Verification items for this drawing (mm, ordinates from the low corner). Round coordinates to 2 decimals unless told otherwise and drop trailing zeros. Write each loop counter-clockwise with the first axis right and the second up, starting at its lowest first coordinate (ties: lowest second). Pieces come first, ordered by that corner, then holes. Notation, with made-up numbers: M 57.25,38 L 74.25,38 A20 ccw 74.25,66 Z; hole C -12.5,-21 d2. An arc over 180 degrees is marked long. Write each question's results on one line, items separated by ' | '.
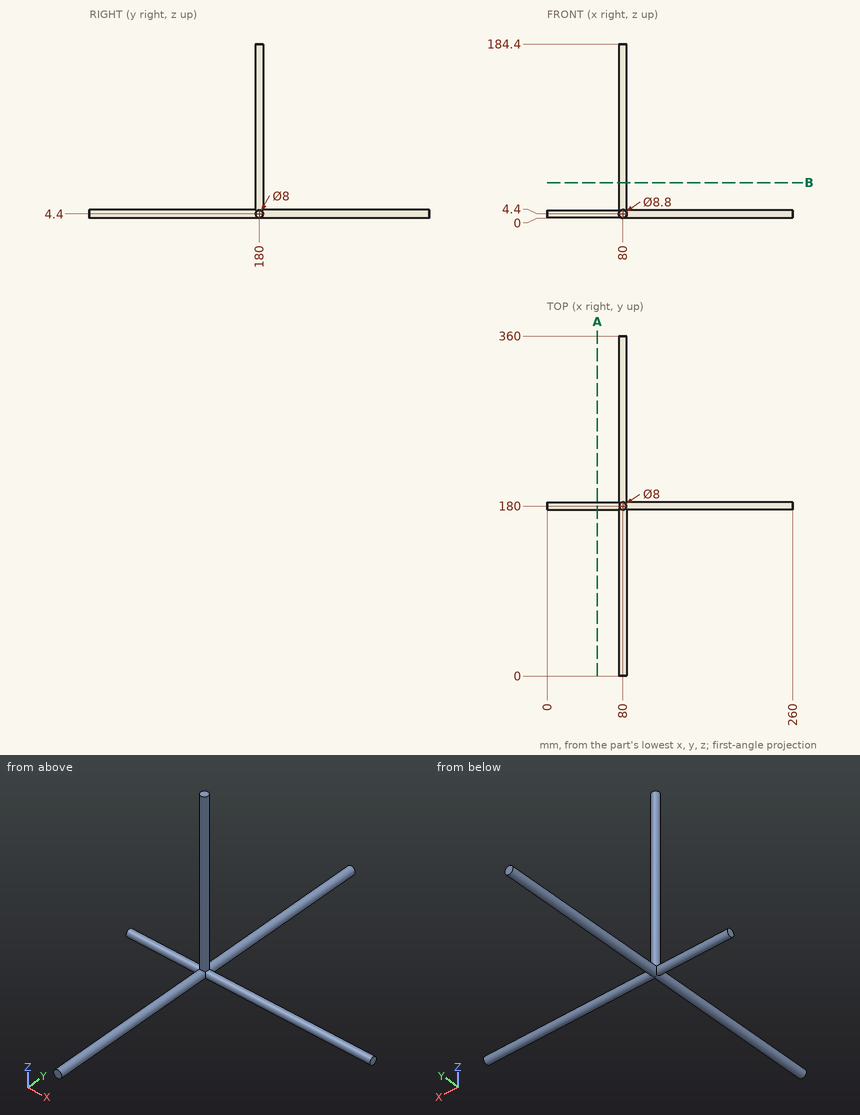
1) Sectioned sample at A-A, the plane x = 53. Record the cut outline in (y, z).
Calculated:
outline: C 180,4.4 d8
2) Material ranges on line 1 (X direction, y = 176.5, z = 92), recorded low to high. Write a range as [from, to].
Calculated:
line 1: x = [78.06, 81.94]
3) Sectioned sample at B-B, the plane z = 37.5. Record the cut outline in (x, y).
Calculated:
outline: C 80,180 d8
4) Depth check by flat-ended pin: P1, Ø1.5, axis at x = 231.5, y = 181.5, coming from the +Z side; P2, Ø10, axis at x = 189.5, y = 169, coming from the -Z side. Enter the tip coordinate at first touch or a pass-through.
Calculated:
P1: stops at z = 8.33 | P2: passes through
